from build123d import *

# Parameters (mm, degrees)
F1_DEPTH = 19.05
F2_DEPTH = 76.2
F3_DEPTH = 20.828
F4_DEPTH = 38.1
F5_DEPTH = 63.5
F6_R     = 50.8
F6_R_2   = 19.05
F7_DEPTH = 31.75
F8_R     = 12.7


with BuildPart() as f1:
    # F0 (on Front) → F1 (new body)
    with BuildSketch(Plane.XZ):
        with BuildLine():
            Line((82.55, 9.525), (101.1525302452, 9.525))
            ThreePointArc((101.1525302452, 9.525), (0, 101.6), (-101.1525302452, 9.525))
            Line((-101.1525302452, 9.525), (-82.55, 9.525))
            Line((-82.55, 9.525), (-82.55, 0))
            Line((-82.55, 0), (-76.2, 0))
            ThreePointArc((-76.2, 0), (-57.1437924233, 50.4086003325), (-9.5063782813, 75.6046875))
            ThreePointArc((-9.5063782813, 75.6046875), (-0.2978018389, 85.7203434321), (9.525, 76.2))
            ThreePointArc((9.525, 76.2), (9.5203434321, 75.9021981611), (9.5063782813, 75.6046875))
            ThreePointArc((9.5063782813, 75.6046875), (57.1437924233, 50.4086003325), (76.2, 0))
            Line((76.2, 0), (82.55, 0))
            Line((82.55, 0), (82.55, 9.525))
        make_face()
        with BuildLine():
            ThreePointArc((-101.1525302452, -9.525), (0, -101.6), (101.1525302452, -9.525))
            Line((101.1525302452, -9.525), (82.55, -9.525))
            Line((82.55, -9.525), (82.55, 0))
            Line((82.55, 0), (76.2, 0))
            ThreePointArc((76.2, 0), (57.1437924233, -50.4086003325), (9.5063782813, -75.6046875))
            ThreePointArc((9.5063782813, -75.6046875), (9.5203434321, -75.9021981611), (9.525, -76.2))
            ThreePointArc((9.525, -76.2), (-0.2978018389, -85.7203434321), (-9.5063782813, -75.6046875))
            ThreePointArc((-9.5063782813, -75.6046875), (-57.1437924233, -50.4086003325), (-76.2, 0))
            Line((-76.2, 0), (-82.55, 0))
            Line((-82.55, 0), (-82.55, -9.525))
            Line((-82.55, -9.525), (-101.1525302452, -9.525))
        make_face()
        with BuildLine():
            ThreePointArc((9.5063782813, -75.6046875), (57.1437924233, -50.4086003325), (76.2, 0))
            Line((76.2, 0), (50.8, 0))
            ThreePointArc((50.8, 0), (0, -50.8), (-50.8, 0))
            Line((-50.8, 0), (-76.2, 0))
            ThreePointArc((-76.2, 0), (-57.1437924233, -50.4086003325), (-9.5063782813, -75.6046875))
            ThreePointArc((-9.5063782813, -75.6046875), (0, -66.675), (9.5063782813, -75.6046875))
        make_face()
        with BuildLine():
            ThreePointArc((-50.8, 0), (0, -50.8), (50.8, 0))
            Line((50.8, 0), (25.4, 0))
            ThreePointArc((25.4, 0), (0, -25.4), (-25.4, 0))
            Line((-25.4, 0), (-50.8, 0))
        make_face()
        with BuildLine():
            Line((25.4, 0), (50.8, 0))
            ThreePointArc((50.8, 0), (0, 50.8), (-50.8, 0))
            Line((-50.8, 0), (-25.4, 0))
            ThreePointArc((-25.4, 0), (0, 25.4), (25.4, 0))
        make_face()
        with BuildLine():
            Line((50.8, 0), (76.2, 0))
            ThreePointArc((76.2, 0), (57.1437924233, 50.4086003325), (9.5063782813, 75.6046875))
            ThreePointArc((9.5063782813, 75.6046875), (0, 66.675), (-9.5063782813, 75.6046875))
            ThreePointArc((-9.5063782813, 75.6046875), (-57.1437924233, 50.4086003325), (-76.2, 0))
            Line((-76.2, 0), (-50.8, 0))
            ThreePointArc((-50.8, 0), (0, 50.8), (50.8, 0))
        make_face()
        with BuildLine():
            ThreePointArc((-19.05, 0), (0, -19.05), (19.05, 0))
            Line((19.05, 0), (0, 0))
            Line((0, 0), (-19.05, 0))
        make_face()
        with BuildLine():
            Line((0, 0), (19.05, 0))
            ThreePointArc((19.05, 0), (0, 19.05), (-19.05, 0))
            Line((-19.05, 0), (0, 0))
        make_face()
        with BuildLine():
            ThreePointArc((9.525, -76.2), (9.5203434321, -75.9021981611), (9.5063782813, -75.6046875))
            ThreePointArc((9.5063782813, -75.6046875), (0, -76.2), (-9.5063782813, -75.6046875))
            ThreePointArc((-9.5063782813, -75.6046875), (-0.2978018389, -85.7203434321), (9.525, -76.2))
        make_face()
        with BuildLine():
            ThreePointArc((-9.5063782813, 75.6046875), (0, 66.675), (9.5063782813, 75.6046875))
            ThreePointArc((9.5063782813, 75.6046875), (0, 76.2), (-9.5063782813, 75.6046875))
        make_face()
        with BuildLine():
            ThreePointArc((-9.5063782813, 75.6046875), (0, 76.2), (9.5063782813, 75.6046875))
            ThreePointArc((9.5063782813, 75.6046875), (9.5203434321, 75.9021981611), (9.525, 76.2))
            ThreePointArc((9.525, 76.2), (-0.2978018389, 85.7203434321), (-9.5063782813, 75.6046875))
        make_face()
        with BuildLine():
            ThreePointArc((-9.5063782813, -75.6046875), (0, -76.2), (9.5063782813, -75.6046875))
            ThreePointArc((9.5063782813, -75.6046875), (0, -66.675), (-9.5063782813, -75.6046875))
        make_face()
        with BuildLine():
            ThreePointArc((-25.4, 0), (0, -25.4), (25.4, 0))
            Line((25.4, 0), (19.05, 0))
            ThreePointArc((19.05, 0), (0, -19.05), (-19.05, 0))
            Line((-19.05, 0), (-25.4, 0))
        make_face()
        with BuildLine():
            Line((19.05, 0), (25.4, 0))
            ThreePointArc((25.4, 0), (0, 25.4), (-25.4, 0))
            Line((-25.4, 0), (-19.05, 0))
            ThreePointArc((-19.05, 0), (0, 19.05), (19.05, 0))
        make_face()
    extrude(amount=-F1_DEPTH)

    # F0 (on Front) → F2 (join)
    with BuildSketch(Plane.XZ):
        with BuildLine():
            Line((0, 0), (19.05, 0))
            ThreePointArc((19.05, 0), (0, 19.05), (-19.05, 0))
            Line((-19.05, 0), (0, 0))
        make_face()
        with BuildLine():
            ThreePointArc((-19.05, 0), (0, -19.05), (19.05, 0))
            Line((19.05, 0), (0, 0))
            Line((0, 0), (-19.05, 0))
        make_face()
    extrude(amount=F2_DEPTH)

    # F0 (on Front) → F3 (join)
    with BuildSketch(Plane.XZ):
        with BuildLine():
            ThreePointArc((-9.5063782813, -75.6046875), (0, -76.2), (9.5063782813, -75.6046875))
            ThreePointArc((9.5063782813, -75.6046875), (0, -66.675), (-9.5063782813, -75.6046875))
        make_face()
        with BuildLine():
            ThreePointArc((9.525, -76.2), (9.5203434321, -75.9021981611), (9.5063782813, -75.6046875))
            ThreePointArc((9.5063782813, -75.6046875), (0, -76.2), (-9.5063782813, -75.6046875))
            ThreePointArc((-9.5063782813, -75.6046875), (-0.2978018389, -85.7203434321), (9.525, -76.2))
        make_face()
        with BuildLine():
            ThreePointArc((-9.5063782813, 75.6046875), (0, 66.675), (9.5063782813, 75.6046875))
            ThreePointArc((9.5063782813, 75.6046875), (0, 76.2), (-9.5063782813, 75.6046875))
        make_face()
        with BuildLine():
            ThreePointArc((-9.5063782813, 75.6046875), (0, 76.2), (9.5063782813, 75.6046875))
            ThreePointArc((9.5063782813, 75.6046875), (9.5203434321, 75.9021981611), (9.525, 76.2))
            ThreePointArc((9.525, 76.2), (-0.2978018389, 85.7203434321), (-9.5063782813, 75.6046875))
        make_face()
    extrude(amount=F3_DEPTH)

    # F0 (on Front) → F4 (join)
    with BuildSketch(Plane.XZ):
        with BuildLine():
            Line((19.05, 0), (25.4, 0))
            ThreePointArc((25.4, 0), (0, 25.4), (-25.4, 0))
            Line((-25.4, 0), (-19.05, 0))
            ThreePointArc((-19.05, 0), (0, 19.05), (19.05, 0))
        make_face()
        with BuildLine():
            ThreePointArc((-25.4, 0), (0, -25.4), (25.4, 0))
            Line((25.4, 0), (19.05, 0))
            ThreePointArc((19.05, 0), (0, -19.05), (-19.05, 0))
            Line((-19.05, 0), (-25.4, 0))
        make_face()
    extrude(amount=-F4_DEPTH)

    # F5 (add): a face of the model
    f5_faces = [f1.faces().sort_by_distance(p)[0] for p in [
        (0, 19.05, 0),
    ]]
    extrude(f5_faces, amount=F5_DEPTH)

    # F6 (on face) → F7 (join)
    with BuildSketch(Plane.XZ.offset(76.2)):
        Circle(F6_R)
        Circle(F6_R_2, mode=Mode.SUBTRACT)
        Circle(F6_R_2)
    extrude(amount=F7_DEPTH)

    # F8
    f8_edges = [f1.edges().sort_by_distance(p)[0] for p in [
        (-50.8, -107.95, 0),
    ]]
    fillet(f8_edges, radius=F8_R)


solid = f1.part
Build history of the part. All positions in model axes, mm. A direction names the side the tool comes from. Round coordinates to 2 decimals unless told otherwise and drop trailing zeros. Write each loop counter-clockwise with the first axis right and the second up, starting at its lowest first coordinate (ties: lowest second). Pieces come first, ordered by that corner, then holes. Notation, with made-up numbers: M 30.5,88 L 60.5,88 A26 cw 60.5,124 Z; hole C 1,-8.75 d3. An arc over 180 degrees is marked long. Answer as a JSON object with one key per item and string values. Group by question number.
(1) Mould opens along Y. For faces 1 (the cylindrical face through (15.12, -37.57, 11.59)), 2 (the flat face through (0, -20.828, -76)), 3 (the flat face through (-1, 0, -21)), 4 (the flat face through (92, 9, -9.525)) say: pulls with the +Y half, pulls with the -Y half, needs draft (parallel to the pull), parting line crosses it, or undercut.
(2) Cut at B-B (z = 0). Give the cut face in (x, y).
(3) Flat gauge pins, fed straight in: pin 1 (5.5 mm diameter, centred on x = -1, z = -79.5, fed in from -Y); pin 2 (3 mm diameter, centred on x = 72, y = 7.5, fed in from -Z); pin 3 (15 mm diameter, centred on x = 88.5, y = 6.5, fed in from +Z); pin 4 (3 mm diameter, centred on y = -39.5, z = 21, fed in from -X). Where does each tip first touch, or does it go through?
(4) Cut at C-C (y = 29). Give the cut face in (x, z), and give its area (3 significant figures).
(5) Which spindle directions (+Z, -Z, +X, -X, +Y, -Y) get a long thin tool onto all of the face, cutting with end or side? Do faces 5 (the flat face through (0, -20.828, 76)), 6 (the flat face through (4, 38.1, 19)), 7 (the flat face through (-92, 9, -9.525)), 8 (the flat face through (22, -76.2, 1)). Say none if no direction does.
(6) Cut at D-D (y = -63.5). Give the cut face in (x, z), and give its area (3 significant figures).
(7) Drill centre lines: L1, parallel to Y at x = -20, z = -4.5; L2, parallel to Y at x = -58.5, z = -61.5; L3, parallel to Y at x = -12.5, z = -23.5. Where is each one in solid material? Low to high.
Responses:
{
 "1": {"face 1": "undercut", "face 2": "pulls with the -Y half", "face 3": "undercut", "face 4": "needs draft"},
 "2": {"outline": "M -82.55,0 L -19.05,0 L -19.05,-76.2 L -50.8,-76.2 L -50.8,-95.25 A12.7 ccw -38.1,-107.95 L 38.1,-107.95 A12.7 ccw 50.8,-95.25 L 50.8,-76.2 L 19.05,-76.2 L 19.05,0 L 82.55,0 L 82.55,19.05 L 25.4,19.05 L 25.4,38.1 L 19.05,38.1 L 19.05,82.55 L -19.05,82.55 L -19.05,38.1 L -25.4,38.1 L -25.4,19.05 L -82.55,19.05 Z"},
 "3": {"pin 1": "stops at y = -20.83", "pin 2": "stops at z = -73.16", "pin 3": "stops at z = 61.33", "pin 4": "passes through"},
 "4": {"outline": "C 0,0 d50.8", "area": "2,030 mm2"},
 "5": {"face 5": "+Z, +X, -X, -Y", "face 6": "+Y", "face 7": "-X, +Y, -Y", "face 8": "none"},
 "6": {"outline": "C 0,0 d38.1", "area": "1,140 mm2"},
 "7": {"L1": "y = -107.95 to -76.2, 0 to 38.1", "L2": "y = 0 to 19.05", "L3": "y = -107.95 to -76.2, 0 to 19.05"}
}
